from build123d import *

# Parameters (mm, degrees)
EXTRUDE_1_DEPTH     = 24
SKETCH_3_W          = 3.392304845
SKETCH_3_H          = 3
SKETCH_4_R          = 7.5
EXTRUDE_2_DEPTH     = 7
SKETCH_5_R          = 5
CUT_EXTRUDE_1_DEPTH = 34.911649916
EXTRUDE_START       = -12
SKETCH_6_R          = 5
SKETCH_6_R_2        = 3.5
EXTRUDE_3_DEPTH     = 12
CHAMFER_1_SIZE      = 5.5
CHAMFER_1_SIZE2     = 1.473720558
SKETCH_7_R          = 11
EXTRUDE_4_DEPTH     = 1.5


with BuildPart() as part:
    # Эскиз1 → Вытянуть1 (new body)
    with BuildSketch(Plane(origin=(0, 0, 0), x_dir=(1, 0, 0), z_dir=(0, 1, 0))):
        Polygon((-5.196152423, 9), (5.196152423, 9), (10.392304845, 0), (5.196152423, -9), (-5.196152423, -9), (-10.392304845, 0), align=None)
    extrude(amount=-EXTRUDE_1_DEPTH)

    # Эскиз2 → Вырез-Повернуть1 (revolve, cut)
    with BuildSketch(Plane.XY, mode=Mode.PRIVATE) as cut_revolve_1_sk:
        with BuildLine():
            Line((8.992304845, -9), (10.392304845, -10))
            Line((10.392304845, -10), (11.881416036, -10))
            Line((11.881416036, -10), (11.881416036, 2.231526293))
            Line((11.881416036, 2.231526293), (6.392304845, 2.231526293))
            Line((6.392304845, 2.231526293), (6.392304845, 0))
            ThreePointArc((6.392304845, 0), (7.430886543, -0.250552945), (8.192304845, -1))
            Line((8.192304845, -1), (8.992304845, -9))
        make_face()
    revolve(cut_revolve_1_sk.sketch.rotate(Axis((0, 9.980849864, 0), (0, -1, 0)), 90), axis=Axis((0, 9.980849864, 0), (0, -1, 0)), mode=Mode.SUBTRACT)

    # Эскиз3 → Вырез-Повернуть2 (revolve, cut)
    with BuildSketch(Plane.XY, mode=Mode.PRIVATE) as cut_revolve_2_sk:
        with Locations((8.696152422, -17.5)):
            Rectangle(SKETCH_3_W, SKETCH_3_H)
    revolve(cut_revolve_2_sk.sketch.rotate(Axis((0, 9.980849864, 0), (0, -1, 0)), 300.000000019), axis=Axis((0, 9.980849864, 0), (0, -1, 0)), mode=Mode.SUBTRACT)

    # Эскиз4 → Вытянуть2 (add)
    with BuildSketch(Plane.XZ.offset(24)):
        with Locations(Location((0, 0, 0), (0, 0, 90))):
            Circle(SKETCH_4_R)
    extrude(amount=EXTRUDE_2_DEPTH)

    # Эскиз5 → Вырез-Вытянуть1 (cut, through all)
    with BuildSketch(Plane.XZ.offset(31)):
        with Locations(Location((0, 0, 0), (0, 0, 270))):
            Circle(SKETCH_5_R)
    extrude(amount=-CUT_EXTRUDE_1_DEPTH, mode=Mode.SUBTRACT)

    # Эскиз6 → Вытянуть3 (add)
    with BuildSketch(Plane(origin=(0, 0, 0), x_dir=(-1, 0, 0), z_dir=(0, 1, 0)).offset(EXTRUDE_START)):
        with Locations(Location((0, 0, 0), (0, 0, 270))):
            Circle(SKETCH_6_R)
        with Locations(Location((0, 0, 0), (0, 0, 90))):
            Circle(SKETCH_6_R_2, mode=Mode.SUBTRACT)
    extrude(amount=EXTRUDE_3_DEPTH)

    # Фаска1
    chamfer_1_edges = [part.edges().sort_by_distance(p)[0] for p in [
        (0, -12, 5),
    ]]
    chamfer_1_side = [part.faces().sort_by_distance(p)[0] for p in [
        (0, -21.5, 5),
    ]]
    chamfer(chamfer_1_edges, length=CHAMFER_1_SIZE, length2=CHAMFER_1_SIZE2, reference=chamfer_1_side[0])

    # Эскиз7 → Вытянуть4 (add)
    with BuildSketch(Plane.XZ.offset(24)):
        with Locations(Location((0, 0, 0), (0, 0, 270))):
            Circle(SKETCH_7_R)
    extrude(amount=EXTRUDE_4_DEPTH)


solid = part.part
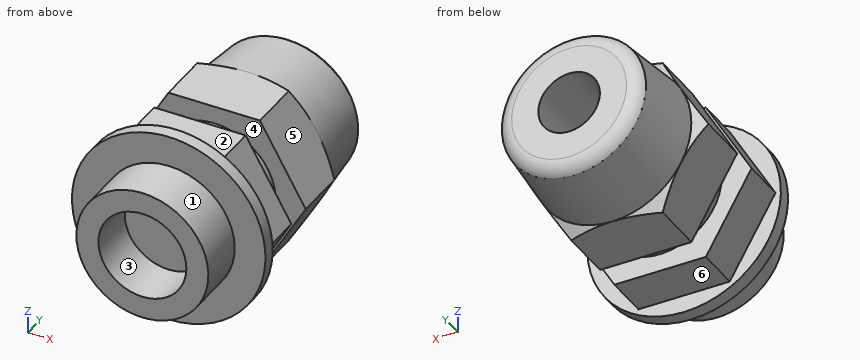
For this review, take the finished solid that the model builds, in its own axes (mm). Face numbers are marked on the shaded views. A direction names the side the tool comes from. Give positions to 0.01 mm unless a question says otherwise; leave off trailing zeros. Order: outer loops, then holes, each group sorted by start corner. A loop starts at its lowest first (then second) coordinate and runs counter-clockwise, first axis right, second up. Notation, with made-up numbers: (-19.75, 8.25) - (17.25, 8.25) arc R3 cw to (17.25, 12.25) - close; hole circle Ø9 at (53.25, -23). An arc over 180 degrees is marked (long way). Answer as a JSON object with one key per item and string values. Group by question number.
Item 1: Wall thickness on line 1 along X through (y, z) = (-20, 0); line 2 along Z through (x, y) = (0, -22.5); line 3 along Y through (x, z) = (-2.25, -2): over which ranges is each line inside the solid? List them lowest first.
Item 2: Machinability: for the marked faces 4, 5 and 6, which of the approach directions +Z, -Z, +X, -X, +Y, -Y give a long, thin tool a straight path to every point of the face, cutting with its end or side? Answer none if there is none.
Item 3: Draft analysis for pull direction Z (two halves, no side actions). For the marked faces 1, 2 and 3, state which applies: pulls with the +Z half, pulls with the -Z half, needs draft (parallel to the pull), parting line crosses it, or undercut.
Item 4: Take a section at A-A on y = -5.5. Give the boundary of the cut face in (x, z), and give its area (3 significant figures).
Item 5: Clearance check with flat-ended pins moving along their axes: pin 1 Ø1.5 at (x, y) = (-1.5, -20.5) entering from -Z; pin 2 Ø3.5 at (x, y) = (-1.5, -13.5) entering from +Z; pin 3 Ø8 at (x, z) = (0, 0) entering from -Y. State where each tip first meets the part, or that it passes through.
Reported:
{
 "1": {"line 1": "-10.39 to -5, 5 to 10.39", "line 2": "-9 to -5, 5 to 9", "line 3": "-25.5 to -24"},
 "2": {"face 4": "none", "face 5": "+Z, +X, +Y", "face 6": "-Z, +X, -X, +Y"},
 "3": {"face 1": "parting line crosses it", "face 2": "pulls with the +Z half", "face 3": "undercut"},
 "4": {"outline": "circle Ø17.28 at (0, 0); hole circle Ø7 at (0, 0)", "area": "196 mm^2"},
 "5": {"pin 1": "z = -9", "pin 2": "z = 9", "pin 3": "y = -25.5"}
}
